Read the model definition and answer for the solid it produces. Units are mm, in the model's axes. Coordinates: 2 decimals unless noted, no trailing zeros. Order: outer loops, then holes, each group sorted by start corner. A loop starts at its lowest first (then second) coordinate and runs counter-clockwise, first axis right, second up. Notation, with made-up numbers: (-31.5, -17) - (1.5, -17) arc R20 cw to (1.5, -2) - close; hole circle Ø1 at (81, 49.25). An arc over 180 degrees is marked (long way). Answer as a JSON object with one key per item and string values. Group by question number.
from build123d import *

# Parameters (mm, degrees)
SKETCH_W        = 40
SKETCH_H        = 96.5
PAD_DEPTH       = 2
SKETCH001_R     = 1.8
SKETCH001_W     = 11.5
SKETCH001_H     = 12.5
SKETCH001_W_2   = 6.5
SKETCH001_H_2   = 8.2
SKETCH001_H_3   = 9.5
SKETCH001_W_3   = 12.4
SKETCH001_H_4   = 20
POCKET_DEPTH    = 5
SKETCH002_W     = 20
SKETCH002_H     = 3
PAD001_DEPTH    = 15
SKETCH003_R     = 1.6
POCKET001_DEPTH = 5


with BuildPart() as part:
    # Sketch → Pad (new body)
    with BuildSketch(Plane.XY):
        Rectangle(SKETCH_W, SKETCH_H)
    extrude(amount=PAD_DEPTH)

    # Sketch001 (on Face6 of Pad) → Pocket (cut)
    with BuildSketch(Plane.XY.offset(2)):
        with Locations((-16.5, 44.95)):
            Circle(SKETCH001_R)
        with Locations((16.5, 44.95)):
            Circle(SKETCH001_R)
        with Locations((-16.5, -44.95)):
            Circle(SKETCH001_R)
        with Locations((16.5, -44.95)):
            Circle(SKETCH001_R)
        with Locations((8.25, -3)):
            Rectangle(SKETCH001_W, SKETCH001_H)
        with Locations((-1.25, 29.95)):
            Rectangle(SKETCH001_W_2, SKETCH001_H_2)
        with Locations((-4.55, -33)):
            Rectangle(SKETCH001_W, SKETCH001_H_3)
        with Locations((12, 24.25)):
            Rectangle(SKETCH001_W_3, SKETCH001_H_4)
    extrude(amount=-POCKET_DEPTH, mode=Mode.SUBTRACT)

    # Sketch002 (on Face4 of Pocket) → Pad001 (join)
    with BuildSketch(Plane(origin=(0, 0, 0), x_dir=(1, 0, 0), z_dir=(0, 0, -1))):
        with Locations((0, -46.75)):
            Rectangle(SKETCH002_W, SKETCH002_H)
    extrude(amount=PAD001_DEPTH)

    # Sketch003 (on Face5 of Pad001) → Pocket001 (cut)
    with BuildSketch(Plane(origin=(0, 48.25, 0), x_dir=(-1, 0, 0), z_dir=(0, 1, 0))):
        with Locations((0, -8.215687)):
            Circle(SKETCH003_R)
    extrude(amount=-POCKET001_DEPTH, mode=Mode.SUBTRACT)


solid = part.part
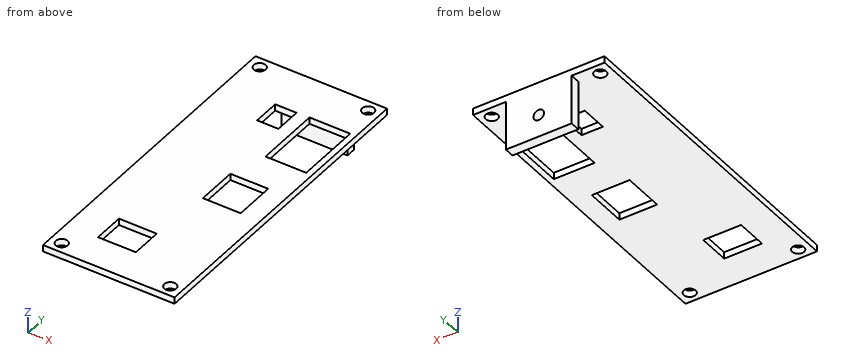
1. A cutting plane is placed at D-D on x = -6. Write down the section's boundary in (y, z), and give its area (3 significant figures).
2. Straight lines are drawn through the part: L1, parallel to Y at x = -16.5, z = 0.75; L2, parallel to Y at x = -7.5, z = -3.5; L3, parallel to Z at x = -16, y = -4. For each, find the intervals that lie inside material, in ascending order.
3. A cutting plane is placed at A-A on x = 16.5. Write down the section's boundary in (y, z), and give its area (3 significant figures).
4. A cutting plane is placed at B-B on y = 33. Write down the section's boundary in (x, z).
5. Given pin 1 (4 mm diameter, centred on x = -16.5, y = 44.95, fed in from -Z); pin 2 (1.5 mm diameter, centred on x = -4, z = -5.5, fed in from -Y), each flat-ended and moving along its own axis, determine where each tip first touches the part or whether it passes through.
6. A cutting plane is placed at C-C on x = 12.5. Write down the section's boundary in (y, z), and give its area (3 significant figures).
Derived:
{
 "1": {"outline": "(-48.25, 0) - (-37.75, 0) - (-37.75, 2) - (-48.25, 2) - close; (-28.25, 0) - (45.25, 0) - (45.25, -15) - (48.25, -15) - (48.25, 2) - (-28.25, 2) - close", "area": "219 mm2"},
 "2": {"L1": "y = -48.25 to -46.75, -43.15 to 43.15, 46.75 to 48.25", "L2": "y = 45.25 to 48.25", "L3": "z = 0 to 2"},
 "3": {"outline": "(-48.25, 0) - (-46.75, 0) - (-46.75, 2) - (-48.25, 2) - close; (-43.15, 0) - (14.25, 0) - (14.25, 2) - (-43.15, 2) - close; (34.25, 0) - (43.15, 0) - (43.15, 2) - (34.25, 2) - close; (46.75, 0) - (48.25, 0) - (48.25, 2) - (46.75, 2) - close", "area": "139 mm2"},
 "4": {"outline": "(-20, 0) - (-4.5, 0) - (-4.5, 2) - (-20, 2) - close; (2, 0) - (5.8, 0) - (5.8, 2) - (2, 2) - close; (18.2, 0) - (20, 0) - (20, 2) - (18.2, 2) - close"},
 "5": {"pin 1": "stops at z = 0", "pin 2": "stops at y = 45.25"},
 "6": {"outline": "(-48.25, 0) - (-9.25, 0) - (-9.25, 2) - (-48.25, 2) - close; (3.25, 0) - (14.25, 0) - (14.25, 2) - (3.25, 2) - close; (34.25, 0) - (48.25, 0) - (48.25, 2) - (34.25, 2) - close", "area": "128 mm2"}
}
